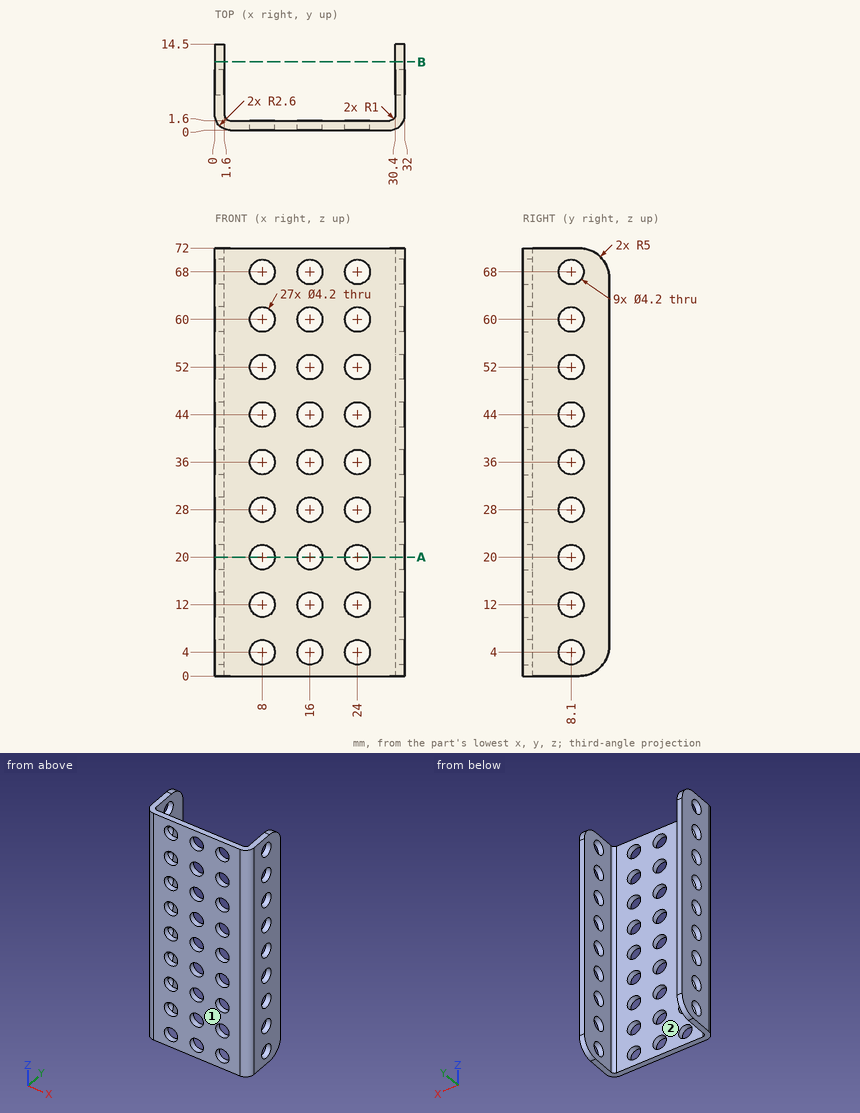
Source: three-view drawing plus pictorial views. Frame: mm from the lowest corner of the part. Give positions to 0.01 mm unless a question says otherwise; leave off trailing zeros. Write each loop counter-clockwise with the first axis right and the second up, starting at its lowest first coordinate (ties: lowest second). Pieces come first, ordered by that corner, then holes. Notation, with made-up numbers: M 3.25,74 L 24.25,74 A22 ccw 24.25,109 Z; hole C -27,-40 d7. An arc over 180 degrees is marked long. Use one line per item in the form item = value.
1. Ray query, L1, parallel to X at y = 0.45, z = 52; L2, parallel to X at y = 4, z = 7; L3, parallel to X at y = 0.55, z = 36. Return the intervals inside material, ascending.
Outcome:
L1 = 1.14 to 5.9, 10.1 to 13.9, 18.1 to 21.9, 26.1 to 30.86
L2 = 0 to 1.6, 30.4 to 32
L3 = 1 to 5.9, 10.1 to 13.9, 18.1 to 21.9, 26.1 to 31
2. Mould query, pull axis X, two halves, no side actions, for the marked faces 1 and 2. Classes: released by +X, released by -X, zero draft, split by the parting line, or undercut.
Outcome:
face_1 = zero draft
face_2 = undercut
3. Cut plane A-A on z = 20. State how many separate pieces and enclosed holes the cut face has, and give its area (3 significant figures).
Outcome:
separate_pieces = 6
enclosed_holes = 0
area = 56.4 mm²
4. Cut plane B-B on y = 11.5. Return loops of the section in (x, z).
Outcome:
outline = M 0,0.42 L 1.6,0.42 L 1.6,71.58 L 0,71.58 Z; M 30.4,0.42 L 32,0.42 L 32,71.58 L 30.4,71.58 Z
5. First-contact query: P1, Ø5, axis at x = 16, z = 60, coming from the -Y side; P2, Ø10, axis at x = 10, z = 36.5, coming from the +Y side; P3, Ø2.5, axis at y = 8.1, z = 4, coming from the +X side. Flat tips, straight axial feed; report the tip coordinate or a pass-through.
Outcome:
P1 = 0
P2 = 1.6
P3 = through
